The model under review builds one solid part; all positions refer to its coordinate system, in mm. Face numbers are marked on the shaded views. A direction names the side the tool comes from. Coordinates: 2 decimals unless noted, no trailing zeros. Order: outer loops, then holes, each group sorted by start corner. A loop starts at its lowest first (then second) coordinate and runs counter-clockwise, first axis right, second up. Notation, with made-up numbers: M -29.75,72.5 L -20.75,72.5 A34 cw -20.75,110.5 Z; hole C 18,17 d5. An arc over 180 degrees is marked long. Answer in a Markdown table with one row per item.
from build123d import *

# Parameters (mm, degrees)
F0_R     = 4.125
F1_DEPTH = 8


with BuildPart() as f1:
    # F0 (on Top) → F1 (new body)
    with BuildSketch(Plane.XY):
        Polygon((8.5, -4.9074772881), (8.5, 4.9074772881), (0, 9.8149545762), (-8.5, 4.9074772881), (-8.5, -4.9074772881), (0, -9.8149545762), align=None)
        Circle(F0_R, mode=Mode.SUBTRACT)
    extrude(amount=F1_DEPTH)

    # F5 (on 3pt) → F6 (revolve, cut)
    with BuildSketch(Plane(origin=(0, 0, 0), x_dir=(0.8660254038, 0.5, 0), z_dir=(0.5, -0.8660254038, 0))):
        Polygon((-15.315942407, 9.5), (-15.315942407, 6.1736737364), (-2.9019237886, 9.5), align=None)
        Polygon((-15.315942407, -1.5), (-2.9019237886, -1.5), (-15.315942407, 1.8263262636), align=None)
    revolve(axis=Axis((0, 0, 4.2626714858), (0, 0, 1)), mode=Mode.SUBTRACT)

    # F7 (on Front) → F8 (revolve)
    with BuildSketch(Plane.XZ):
        with BuildLine():
            Line((-8.34139258, 8), (-4.25, 8))
            Line((-4.25, 8), (-4.25, 10))
            Line((-4.25, 10), (-5.6916165822, 10))
            ThreePointArc((-5.6916165822, 10), (-6.6151138087, 9.7740216664), (-7.3299206708, 9.1471528727))
            Line((-7.3299206708, 9.1471528727), (-8.0137317623, 8.1705694255))
            ThreePointArc((-8.0137317623, 8.1705694255), (-8.1566931347, 8.0451956667), (-8.34139258, 8))
        make_face()
    revolve(axis=Axis((0, 0, 4.2626714858), (0, 0, 1)))


solid = f1.part
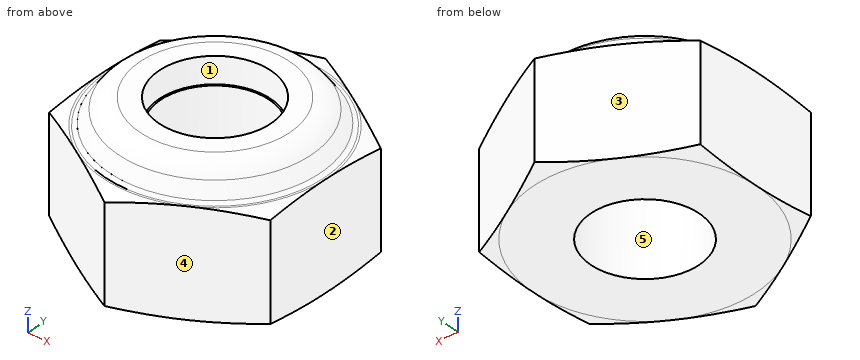
(1) To check wall thickness, follow line 1 (Y direction, x = -2, z = 8.5); line 2 (X direction, y = 1.5, z = 4.5); line 3 (X direction, y = -5, z = 2.5). State the ranges of each line that lie inside material, in increasing order. Write a range as [from, to].
Report:
| item | result |
|---|---|
| line 1 | [-7.52, -3.75], [3.75, 7.52] |
| line 2 | [-8.5, -3.84], [3.84, 8.5] |
| line 3 | [-8.34, 8.34] |
(2) The part is to be moulded in two halves that separate along Y. For the marked faces 3, 4 and 5, say which applies: +Y half, -Y half, draft (parallel to the pull), parting line (faces both ways), or undercut.
Report:
| item | result |
|---|---|
| face 3 | +Y half |
| face 4 | -Y half |
| face 5 | undercut |
(3) Take a section at A-A (z = 4.5). Write out the cut boundary in (x, y) (3 decimals).
Report:
| item | result |
|---|---|
| outline | M -8.5,-4.907 L 0,-9.815 L 8.5,-4.907 L 8.5,4.907 L 0,9.815 L -8.5,4.907 Z; hole C 0,0 d8.25 |
(4) Machinability: for the marked faces 1 and 2, which of the approach directions +Z, -Z, +X, -X, +Y, -Y give a long, thin tool a straight path to every point of the face, cutting with its end or side? Answer none if there is none.
Report:
| item | result |
|---|---|
| face 1 | +Z |
| face 2 | +Z, -Z, +X, +Y, -Y |
(5) Insertion check: P1, Ø2, axis at x = -0.5, z = 3.5, coming from the +Y side; P2, Ø1, axis at x = 5.5, z = 4, coming from the +Y side. Each pin has a flat end and moves straight along its axis. Give the tip position at first contact, or say it passes through.
Report:
| item | result |
|---|---|
| P1 | y = 9.81 |
| P2 | y = 6.93 |
